For this review, use the dimensioned drawing (mm, ordinates from the lowest corner) and the shaded views. A direction names the side the tool comes from. Give positions to 0.01 mm unless a question says otherwise; leave off trailing zeros. Order: outer loops, then holes, each group sorted by start corner. A loop starts at its lowest first (then second) coordinate and runs counter-clockwise, first axis right, second up. Notation, with made-up numbers: (52, 29.5) -> (64, 29.5) arc R31 ccw to (64, 55.5) -> close; hole circle Ø3 at (47.5, 14). An arc over 180 degrees is marked (long way). Answer as a JSON object with one key per item and string values. Group by question number.
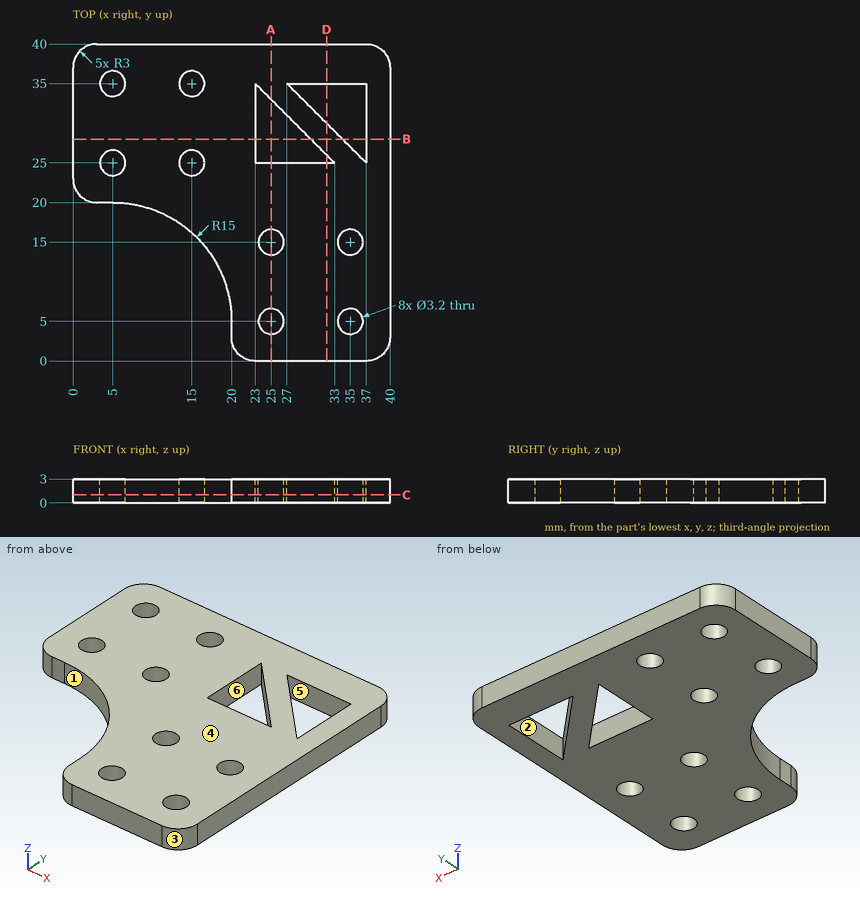
1. Take a section at C-C on z = 1. State how many separate pieces and enclosed holes the cut face has, plus the area to 3 significant figures.
2. Take a section at B-B on y = 28. Give the boundary of the cut face in (x, z), plus the area to 3 significant figures.
3. Take a section at D-D on x = 32. Give the boundary of the cut face in (y, z), plus the area to 3 significant figures.
4. Take a section at A-A on x = 25. Give the boundary of the cut face in (y, z), plus the area to 3 significant figures.
5. For probe 1 along X at (y, z) = (25.5, 0.95); probe 2 along X at (y, z) = (30.5, 1); probe 3 along Y at (x, z) = (30, 0.6), list the stretches that pass through material, from the lowest coordinate up. Write a range as [from, to].
6. For pin 1 (1.9 mm diameter, centred on x = 15, y = 35, fed in from -Z); pin 2 (1.5 mm diameter, centred on y = 17, z = 1.5, fed in from -X); pin 3 (1.6 mm diameter, centred on x = 4, z = 2, fed in from -Y), all flat-tipped, find the tip position at first contact; note any pin that passes through.
7. Draft analysis for pull direction Y (two halves, no side actions). For the marked faces 3, 4, 5 and 6, state which applies: pulls with the +Y half, pulls with the -Y half, needs draft (parallel to the pull), parting line crosses it, or undercut.
8. Machinability: for the marked faces 1 and 2, which of the approach directions +Z, -Z, +X, -X, +Y, -Y give a long, thin tool a straight path to every point of the face, cutting with its end or side? Answer none if there is none.
Checks:
{
 "1": {"separate pieces": "1", "enclosed holes": "10", "area": "1,070 mm2"},
 "2": {"outline": "(0, 0) -> (23, 0) -> (23, 3) -> (0, 3) -> close; (30, 0) -> (34, 0) -> (34, 3) -> (30, 3) -> close; (37, 0) -> (40, 0) -> (40, 3) -> (37, 3) -> close", "area": "90.0 mm2"},
 "3": {"outline": "(0, 0) -> (25, 0) -> (25, 3) -> (0, 3) -> close; (26, 0) -> (30, 0) -> (30, 3) -> (26, 3) -> close; (35, 0) -> (40, 0) -> (40, 3) -> (35, 3) -> close", "area": "102 mm2"},
 "4": {"outline": "(0, 0) -> (3.4, 0) -> (3.4, 3) -> (0, 3) -> close; (6.6, 0) -> (13.4, 0) -> (13.4, 3) -> (6.6, 3) -> close; (16.6, 0) -> (25, 0) -> (25, 3) -> (16.6, 3) -> close; (33, 0) -> (40, 0) -> (40, 3) -> (33, 3) -> close", "area": "76.8 mm2"},
 "5": {"probe 1": "x = [0, 3.48], [6.52, 13.48], [16.52, 23], [32.5, 36.5], [37, 40]", "probe 2": "x = [0, 23], [27.5, 31.5], [37, 40]", "probe 3": "y = [0, 25], [28, 32], [35, 40]"},
 "6": {"pin 1": "passes through", "pin 2": "stops at x = 12.9", "pin 3": "stops at y = 20"},
 "7": {"face 3": "pulls with the -Y half", "face 4": "needs draft", "face 5": "undercut", "face 6": "undercut"},
 "8": {"face 1": "+Z, -Z, -X, -Y", "face 2": "+Z, -Z"}
}
